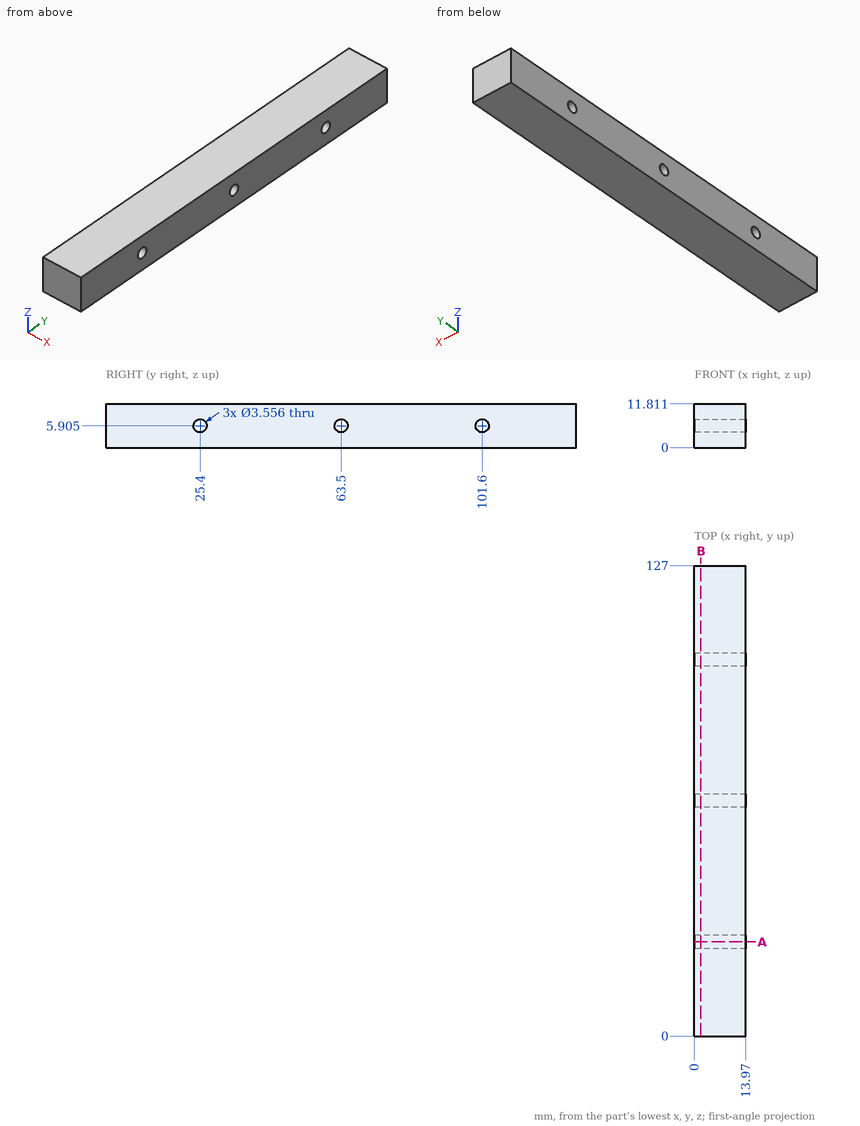
Geometry check sheet. Reference: drawing and pictorial views, mm from the part's lowest x, y, z. Give positions to 0.01 mm unless a question says otherwise; leave off trailing zeros. Write each loop counter-clockwise with the first axis right and the second up, starting at its lowest first coordinate (ties: lowest second). Pieces come first, ordered by that corner, then holes.
Item 1: Cross-section at A-A (y = 25.4). Enter the section's corners in (x, z).
Item 2: Cross-section at B-B (x = 1.75). Enter the section's corners in (y, z) (1 decimal), and give its area (3 significant figures).
Item 3: Scan lines: L1, parallel to Y at x = 10, z = 5.5; L2, parallel to Y at x = 9.5, z = 4.5; L3, parallel to Z at x = 4.75, y = 101.6. Record each from-to range of solid material in increasing order.
Report:
1. outline: (0, 0) - (13.97, 0) - (13.97, 4.13) - (0, 4.13) - close; (0, 7.68) - (13.97, 7.68) - (13.97, 11.81) - (0, 11.81) - close
2. outline: (0, 0) - (127, 0) - (127, 11.8) - (0, 11.8) - close; hole circle Ø3.6 at (25.4, 5.9); hole circle Ø3.6 at (63.5, 5.9); hole circle Ø3.6 at (101.6, 5.9)
2. area: 1,470 mm2
3. L1: y = 0 to 23.67, 27.13 to 61.77, 65.23 to 99.87, 103.33 to 127
3. L2: y = 0 to 24.31, 26.49 to 62.41, 64.59 to 100.51, 102.69 to 127
3. L3: z = 0 to 4.13, 7.68 to 11.81
